Verification items for this drawing (mm, ordinates from the low corner). A direction names the side the tool comes from. Coordinates: 2 decimals unless noted, no trailing zeros. Order: outer loops, then holes, each group sorted by start corner. A loop starts at its lowest first (then second) coordinate and runs counter-clockwise, first axis right, second up. Notation, with made-up numbers: (67.25, -31) -> (71.25, -31) arc R19 cw to (71.25, 1) -> close; hole circle Ø2 at (39, 62.25). An arc over 180 degrees is marked (long way). Answer as CSV lines item,"result". Start each with the question number.
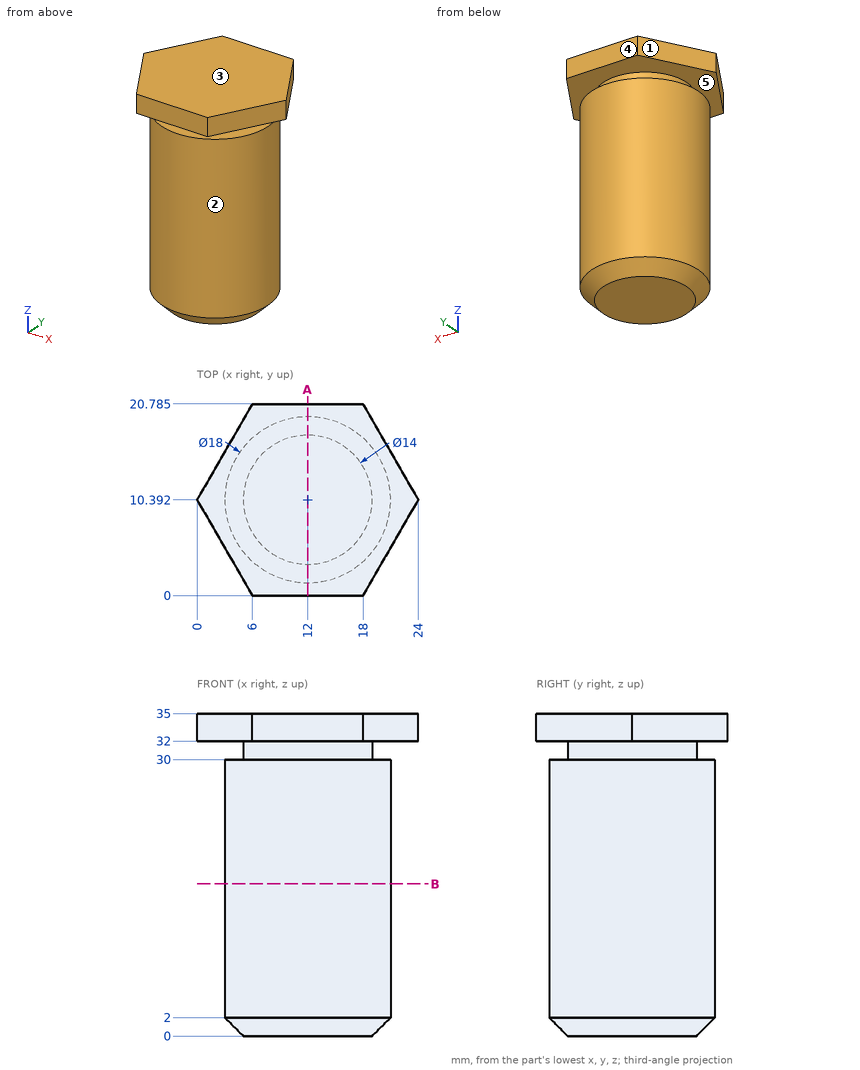
Q1. Access from +Z, -Z, +X, -X, +Y, -Y to the whole of each face (thin tool, end or side, straight path). Record for the marked faces 1 and 2.
Q2. Release check for a two-part mould opening along Z. For the marked faces 3, 4 and 5 record: released by +Z, released by -Z, zero draft, split by the parting line, or undercut.
Q3. Go/stop test with flat-tipped pins: pin 1 Ø6 at (y, z) = (7.5, 18.5) entering from +X; pin 2 Ø8 at (y, z) = (11, 10) entering from -X; pin 3 Ø5 at (x, y) = (7, 10.5) entering from -Z; pin 4 Ø8 at (y, z) = (17, 8) entering from -X. Record where each tip stops, or that it passes through.
Q4. Sectioned sample at A-A, the plane x = 12. Record the cut outline in (y, z) (1 decimal), then the cut area to 3 significant figures.
Q5. Sectioned sample at B-B, the plane z = 16.5. Record the cut outline in (x, y).
Q6. Thickness scan on L1, parallel to Z at x = 18.25, y = 16.75 (1 decimal); L2, parallel to Z at x = 19.25, y = 17.75; L3, parallel to Z at x = 20.5, y = 10.5. Record the ranges inside material, lowest first.
Geometry results:
1,face 1,"+Z, -Z, -X, +Y"
1,face 2,"-Z"
2,face 3,"released by +Z"
2,face 4,"zero draft"
2,face 5,"undercut"
3,pin 1,"stops at x = 21"
3,pin 2,"stops at x = 3"
3,pin 3,"stops at z = 0"
3,pin 4,"stops at x = 3.39"
4,outline,"(0, 32) -> (3.4, 32) -> (3.4, 30) -> (1.4, 30) -> (1.4, 2) -> (3.4, 0) -> (17.4, 0) -> (19.4, 2) -> (19.4, 30) -> (17.4, 30) -> (17.4, 32) -> (20.8, 32) -> (20.8, 35) -> (0, 35) -> close"
4,area,"626 mm^2"
5,outline,"circle Ø18 at (12, 10.39)"
6,L1,"z = 1.9 to 30, 32 to 35"
6,L2,"z = 32 to 35"
6,L3,"z = 1.5 to 30, 32 to 35"
